from build123d import *

# Parameters (mm, degrees)
SKETCH1_R           = 3
BOSS_EXTRUDE1_DEPTH = 50
SKETCH2_R           = 5.8
BOSS_EXTRUDE2_DEPTH = 4.3
FILLET1_R           = 1


with BuildPart() as part:
    # Sketch1 → Boss-Extrude1 (new body)
    with BuildSketch(Plane(origin=(0, 0, 0), x_dir=(1, 0, 0), z_dir=(0, 1, 0))):
        with Locations(Location((0, 0, 0), (0, 0, 270))):  # turned: the seam where the file's is
            Circle(SKETCH1_R)
    extrude(amount=BOSS_EXTRUDE1_DEPTH)

    # Sketch2 → Boss-Extrude2 (add)
    with BuildSketch(Plane(origin=(0, 50, 0), x_dir=(1, 0, 0), z_dir=(0, 1, 0))):
        with Locations(Location((0, 0, 0), (0, 0, 270))):  # turned: the seam where the file's is
            Circle(SKETCH2_R)
    extrude(amount=BOSS_EXTRUDE2_DEPTH)

    # Fillet1
    fillet1_edges = [part.edges().sort_by_distance(p)[0] for p in [
        (0, 50, -5.8),
        (0, 54.3, -5.8),
    ]]
    fillet(fillet1_edges, radius=FILLET1_R)


solid = part.part
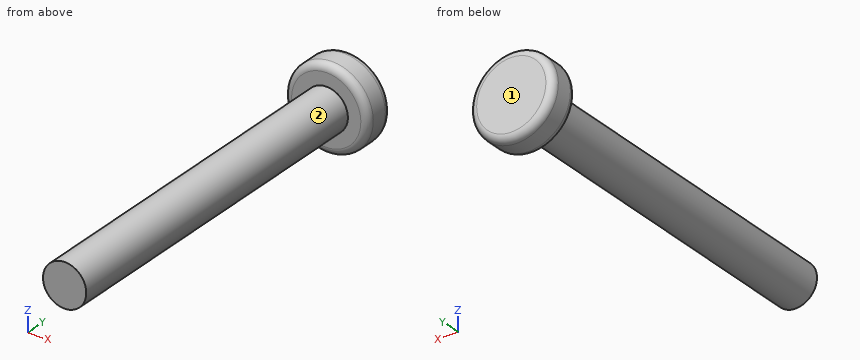
Model file for the job. Use its own axes, mm. Face numbers are marked on the shaded views. A direction names the side the tool comes from. Coordinates: 2 decimals unless noted, no trailing zeros. Write each loop counter-clockwise with the first axis right and the second up, starting at its lowest first coordinate (ties: lowest second). Pieces come first, ordered by that corner, then holes. Notation, with made-up numbers: (16.5, -9.5) -> (53.5, -9.5) arc R23 ccw to (53.5, 4.5) -> close; hole circle Ø8 at (-30, -10.5). An arc over 180 degrees is marked (long way). One line per item, written item: value. Start each with the question number.
1) Slice it at C-C on y = 18. Write the cut outline in (x, z), then the cut area to 3 significant figures.
2) Probe probe 1 along Y at (x, z) = (-2.25, -4.25); probe 2 along X at (y, z) = (18, 2.5); probe 3 along Z at (x, y) = (-0.5, 22). List the from-to ranges inside material, lowest first.
3) Which spindle directions (+Z, -Z, +X, -X, +Y, -Y) get a long thin tool onto all of the face, cutting with end or side? Do the marked faces 1 and 2. Say none if no direction does.
4) Slice it at A-A on z = 0. Write the cut outline in (x, y).
5) Flat gauge pins, fed straight in: pin 1 Ø5 at (y, z) = (25, -0.5) entering from -X; pin 2 Ø2 at (x, y) = (2, 13.5) entering from -Z; pin 3 Ø3 at (x, y) = (0, 24) entering from -Z. Where does each tip first touch, or does it go through?
6) Slice it at B-B on x = 0. Write the cut outline in (y, z), then the cut area to 3 significant figures.
Answers follow:
1. outline: circle Ø6 at (0, 0)
1. area: 28.3 mm2
2. probe 1: 50 to 54.3
2. probe 2: -1.66 to 1.66
2. probe 3: -2.96 to 2.96
3. face 1: +Z, -Z, +X, -X, +Y
3. face 2: -Y
4. outline: (-5.8, 51) arc R1 ccw to (-4.8, 50) -> (-3, 50) -> (-3, 0) -> (3, 0) -> (3, 50) -> (4.8, 50) arc R1 ccw to (5.8, 51) -> (5.8, 53.3) arc R1 ccw to (4.8, 54.3) -> (-4.8, 54.3) arc R1 ccw to (-5.8, 53.3) -> close
5. pin 1: x = -3
5. pin 2: z = -2.83
5. pin 3: z = -3
6. outline: (0, -3) -> (50, -3) -> (50, -4.8) arc R1 ccw to (51, -5.8) -> (53.3, -5.8) arc R1 ccw to (54.3, -4.8) -> (54.3, 4.8) arc R1 ccw to (53.3, 5.8) -> (51, 5.8) arc R1 ccw to (50, 4.8) -> (50, 3) -> (0, 3) -> close
6. area: 349 mm2
